Check sheet for the drawn part. Datum: minimum x, y, z corner. Units: mm. A direction names the side the tool comes from. Coordinates: 2 decimals unless noted, no trailing zeros. Loops run counter-clockwise (first coordinate to the right, second up) from the corner with the lowest first, then second, coordinate; pieces in that order, holes last. Notation, with made-up numbers: (38, -8.75) -> (73, -8.75) arc R16 cw to (73, -4.75) -> close; hole circle Ø8 at (77, 76). An arc over 180 degrees is marked (long way). Use CSV: the item, a comma, the result in double quotes. Start each with the question number.
1. Gauge pin test, flat ends, axial feed: pin 1 (2.5 mm diameter, centred on x = 6, y = 4, fed in from -Z); pin 2 (3 mm diameter, centred on x = 5, y = 3.5, fed in from +Z); pin 3 (1 mm diameter, centred on x = 7, y = 3, fed in from +Z). Record the tip position at first contact, or that the pin passes through.
2. Release check for a two-part mould opening along X. For the marked faces 5, 6 and 7 record: pulls with the +X half, pulls with the -X half, needs draft (parallel to the pull), parting line crosses it, or undercut.
3. Sectioned sample at C-C, the plane y = 3.6. Record the cut outline in (x, z).
4. Sectioned sample at B-B, the plane z = 1.5. Record the cut outline in (x, y), and give its area (3 significant figures).
5. Thickness scan on L1, parallel to Z at x = 3, y = 3.3; L2, parallel to X at y = 4.9, z = 1.9; L3, parallel to X at y = 2.6, z = 1.3. Record the ranges inside material, lowest first.
6. Sectioned sample at D-D, the plane z = 0.2. Record the cut outline in (x, y), and give its area (3 significant figures).
7. Set-up check for the marked faces 1, 2, 3 and 4: record each of +Z, -Z, +X, -X, +Y, -Y from which the full face is reachable in a straight line by a thin tool's end or side.
8. Sectioned sample at A-A, the plane x = 3. Record the cut outline in (y, z).
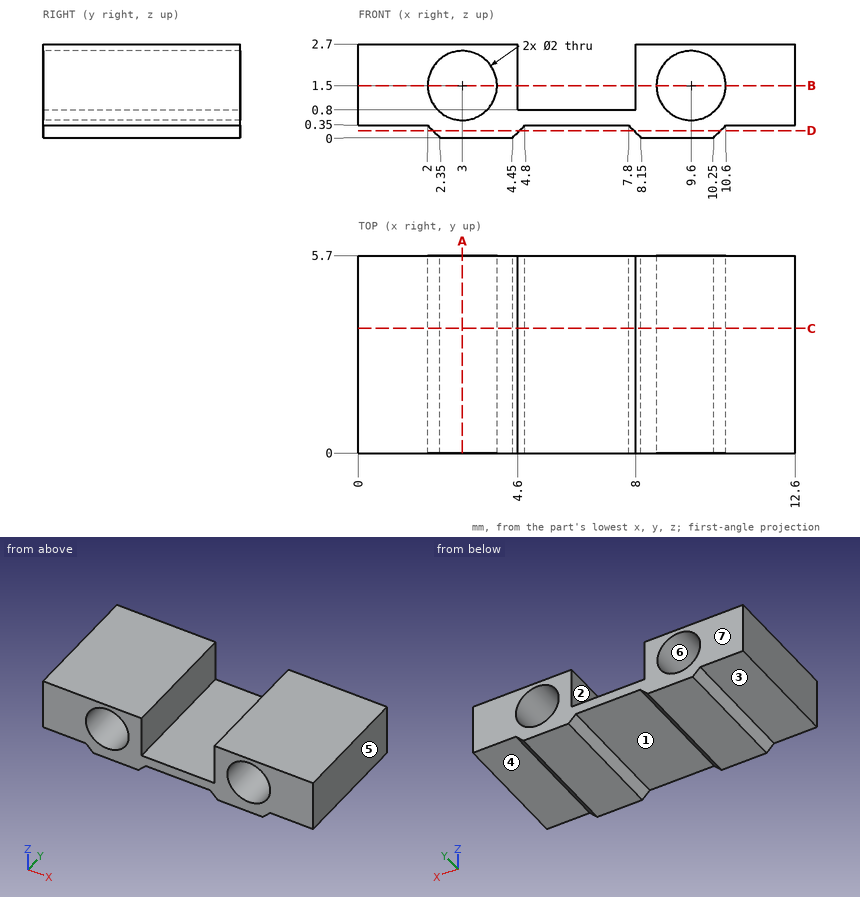
Completed:
1,pin 1,"z = 0.3"
1,pin 2,"z = 2.7"
1,pin 3,"z = 0.8"
2,face 5,"pulls with the +X half"
2,face 6,"undercut"
2,face 7,"needs draft"
3,outline,"(0, 0.35) -> (2, 0.35) -> (2.35, 0) -> (4.45, 0) -> (4.8, 0.35) -> (7.8, 0.35) -> (8.15, 0) -> (10.25, 0) -> (10.6, 0.35) -> (12.6, 0.35) -> (12.6, 2.7) -> (8, 2.7) -> (8, 0.8) -> (4.6, 0.8) -> (4.6, 2.7) -> (0, 2.7) -> close; hole circle Ø2 at (3, 1.5); hole circle Ø2 at (9.6, 1.5)"
4,outline,"(0, 0) -> (2, 0) -> (2, 5.7) -> (0, 5.7) -> close; (4, 0) -> (4.6, 0) -> (4.6, 5.7) -> (4, 5.7) -> close; (8, 0) -> (8.6, 0) -> (8.6, 5.7) -> (8, 5.7) -> close; (10.6, 0) -> (12.6, 0) -> (12.6, 5.7) -> (10.6, 5.7) -> close"
4,area,"29.6 mm²"
5,L1,"0 to 0.5, 2.5 to 2.7"
5,L2,"0 to 2.08, 3.92 to 4.6, 8 to 8.68, 10.52 to 12.6"
5,L3,"0 to 2.02, 3.98 to 4.6, 8 to 8.62, 10.58 to 12.6"
6,outline,"(2.15, 0) -> (4.65, 0) -> (4.65, 5.7) -> (2.15, 5.7) -> close; (7.95, 0) -> (10.45, 0) -> (10.45, 5.7) -> (7.95, 5.7) -> close"
6,area,"28.5 mm²"
7,face 1,"-Z, +Y, -Y"
7,face 2,"+Z, +Y, -Y"
7,face 3,"-Z, -X, +Y, -Y"
7,face 4,"-Z, +X, +Y, -Y"
8,outline,"(0, 0) -> (5.7, 0) -> (5.7, 0.5) -> (0, 0.5) -> close; (0, 2.5) -> (5.7, 2.5) -> (5.7, 2.7) -> (0, 2.7) -> close"
